```python
from build123d import *

# Parameters (mm, degrees)
F0_R     = 16.3195
F0_R_2   = 0.635
F1_DEPTH = 2.54
F0_R_3   = 20.1295
F2_DEPTH = 19.05


with BuildPart() as f1:
    # F0 (on Top) → F1 (new body)
    with BuildSketch(Plane.XY):
        Circle(F0_R)
        with Locations((-10.644357, -10.906661)):
            Circle(F0_R_2, mode=Mode.SUBTRACT)
        with Locations((-5.567701, -14.186554)):
            Circle(F0_R_2, mode=Mode.SUBTRACT)
        with Locations((-14.003354, -6.013625)):
            Circle(F0_R_2, mode=Mode.SUBTRACT)
        with Locations((-7.184205, -7.184205)):
            Circle(F0_R_2, mode=Mode.SUBTRACT)
        with Locations((-3.888064, -9.386616)):
            Circle(F0_R_2, mode=Mode.SUBTRACT)
        with Locations((-9.388233, -3.884157)):
            Circle(F0_R_2, mode=Mode.SUBTRACT)
        with Locations((-3.592102, -3.592102)):
            Circle(F0_R_2, mode=Mode.SUBTRACT)
        with Locations((-1.944032, -4.693308)):
            Circle(F0_R_2, mode=Mode.SUBTRACT)
        with Locations((-4.694117, -1.942079)):
            Circle(F0_R_2, mode=Mode.SUBTRACT)
        with Locations((0, -15.24)):
            Circle(F0_R_2, mode=Mode.SUBTRACT)
        with Locations((0, -12.7)):
            Circle(F0_R_2, mode=Mode.SUBTRACT)
        with Locations((0, -10.16)):
            Circle(F0_R_2, mode=Mode.SUBTRACT)
        with Locations((6.013625, -14.003354)):
            Circle(F0_R_2, mode=Mode.SUBTRACT)
        with Locations((10.543106, -10.289545)):
            Circle(F0_R_2, mode=Mode.SUBTRACT)
        with Locations((3.982214, -9.347062)):
            Circle(F0_R_2, mode=Mode.SUBTRACT)
        with Locations((0, -7.184205)):
            Circle(F0_R_2, mode=Mode.SUBTRACT)
        with Locations((0, -5.08)):
            Circle(F0_R_2, mode=Mode.SUBTRACT)
        with Locations((7.184205, -7.184205)):
            Circle(F0_R_2, mode=Mode.SUBTRACT)
        with Locations((1.944032, -4.693308)):
            Circle(F0_R_2, mode=Mode.SUBTRACT)
        with Locations((3.592102, -3.592102)):
            Circle(F0_R_2, mode=Mode.SUBTRACT)
        with Locations((4.693308, -1.944032)):
            Circle(F0_R_2, mode=Mode.SUBTRACT)
        with Locations((9.386616, -3.888064)):
            Circle(F0_R_2, mode=Mode.SUBTRACT)
        with Locations((14.186554, -5.567701)):
            Circle(F0_R_2, mode=Mode.SUBTRACT)
        with Locations((-15.24, 0)):
            Circle(F0_R_2, mode=Mode.SUBTRACT)
        with Locations((-12.7, 0)):
            Circle(F0_R_2, mode=Mode.SUBTRACT)
        with Locations((-10.16, 0)):
            Circle(F0_R_2, mode=Mode.SUBTRACT)
        with Locations((-14.124854, 5.548119)):
            Circle(F0_R_2, mode=Mode.SUBTRACT)
        with Locations((-7.184205, 0)):
            Circle(F0_R_2, mode=Mode.SUBTRACT)
        with Locations((-5.08, 0)):
            Circle(F0_R_2, mode=Mode.SUBTRACT)
        with Locations((-9.386616, 3.888064)):
            Circle(F0_R_2, mode=Mode.SUBTRACT)
        with Locations((-4.693308, 1.944032)):
            Circle(F0_R_2, mode=Mode.SUBTRACT)
        with Locations((-3.592102, 3.592102)):
            Circle(F0_R_2, mode=Mode.SUBTRACT)
        with Locations((-1.944032, 4.693308)):
            Circle(F0_R_2, mode=Mode.SUBTRACT)
        with Locations((-7.184205, 7.184205)):
            Circle(F0_R_2, mode=Mode.SUBTRACT)
        with Locations((-3.888064, 9.386616)):
            Circle(F0_R_2, mode=Mode.SUBTRACT)
        with Locations((-10.906661, 10.644357)):
            Circle(F0_R_2, mode=Mode.SUBTRACT)
        with Locations((-6.013625, 14.003354)):
            Circle(F0_R_2, mode=Mode.SUBTRACT)
        Circle(F0_R_2, mode=Mode.SUBTRACT)
        with Locations((1.944032, 4.693308)):
            Circle(F0_R_2, mode=Mode.SUBTRACT)
        with Locations((3.592102, 3.592102)):
            Circle(F0_R_2, mode=Mode.SUBTRACT)
        with Locations((5.08, 0)):
            Circle(F0_R_2, mode=Mode.SUBTRACT)
        with Locations((7.184205, 0)):
            Circle(F0_R_2, mode=Mode.SUBTRACT)
        with Locations((5.04853, 2.09117)):
            Circle(F0_R_2, mode=Mode.SUBTRACT)
        with Locations((0, 5.08)):
            Circle(F0_R_2, mode=Mode.SUBTRACT)
        with Locations((0, 7.184205)):
            Circle(F0_R_2, mode=Mode.SUBTRACT)
        with Locations((3.888064, 9.386616)):
            Circle(F0_R_2, mode=Mode.SUBTRACT)
        with Locations((7.184205, 7.184205)):
            Circle(F0_R_2, mode=Mode.SUBTRACT)
        with Locations((10.16, 0)):
            Circle(F0_R_2, mode=Mode.SUBTRACT)
        with Locations((12.7, 0)):
            Circle(F0_R_2, mode=Mode.SUBTRACT)
        with Locations((10.09706, 4.182339)):
            Circle(F0_R_2, mode=Mode.SUBTRACT)
        with Locations((15.24, 0)):
            Circle(F0_R_2, mode=Mode.SUBTRACT)
        with Locations((14.003354, 6.013625)):
            Circle(F0_R_2, mode=Mode.SUBTRACT)
        with Locations((0, 10.16)):
            Circle(F0_R_2, mode=Mode.SUBTRACT)
        with Locations((0, 12.7)):
            Circle(F0_R_2, mode=Mode.SUBTRACT)
        with Locations((5.567701, 14.186554)):
            Circle(F0_R_2, mode=Mode.SUBTRACT)
        with Locations((0, 15.24)):
            Circle(F0_R_2, mode=Mode.SUBTRACT)
        with Locations((10.644357, 10.906661)):
            Circle(F0_R_2, mode=Mode.SUBTRACT)
    extrude(amount=F1_DEPTH)

    # F0 (on Top) → F2 (join)
    with BuildSketch(Plane.XY):
        Circle(F0_R_3)
        Circle(F0_R, mode=Mode.SUBTRACT)
    extrude(amount=F2_DEPTH)


solid = f1.part
```
Check sheet for the modelled part. Datum: model origin and axes. Units: mm. Give positions to 0.01 mm unless a question says otherwise; leave off trailing zeros. Loops run counter-clockwise (first coordinate to the right, second up) from the corner with the lowest first, then second, coordinate; pieces in that order, holes last. Notation, with made-up numbers: M 67,63 L 104,63 A17 ccw 104,70 Z; hole C 13,-8.75 d9. An arc over 180 degrees is marked long. Answer as CSV lines item,"result".
Item 1: Sectioned sample at A-A, the plane x = -2. Enter the section's corners in (y, z), then the cut area to 3 significant figures.
Reply:
outline,"M -20.03,0 L -5.33,0 L -5.33,2.54 L -16.2,2.54 L -16.2,19.05 L -20.03,19.05 Z; M -4.06,0 L 4.06,0 L 4.06,2.54 L -4.06,2.54 Z; M 5.33,0 L 20.03,0 L 20.03,19.05 L 16.2,19.05 L 16.2,2.54 L 5.33,2.54 Z"
area,"222 mm^2"
Item 2: Sectioned sample at B-B, the plane y = -12.7. Enter the section's corners in (x, z) (3 decimals).
Reply:
outline,"M -15.618,0 L -0.635,0 L -0.635,2.54 L -10.249,2.54 L -10.249,19.05 L -15.618,19.05 Z; M 0.635,0 L 15.618,0 L 15.618,19.05 L 10.249,19.05 L 10.249,2.54 L 0.635,2.54 Z"
Item 3: Scan lines: L1, parallel to Y at x = -10.16, z = 1.4 (3 decimals); L2, parallel to Y at x = 13.5, z = 4.5; L3, parallel to X at y = -0.5, z = 6.75. Record each from-to range of solid material in increasing order.
Reply:
L1,"-17.377 to -11.317, -10.496 to -0.635, 0.635 to 17.377"
L2,"-14.93 to -9.17, 9.17 to 14.93"
L3,"-20.12 to -16.31, 16.31 to 20.12"
Item 4: Depth check by flat-ended pin: pin 1 Ø1.5 at (x, y) = (-7.18, -7.18) entering from +Z; pin 2 Ø5 at (x, z) = (5, 3.5) entering from +Y; pin 3 Ø1 at (y, z) = (11, 6) entering from -X. Enter the tip coordinate at first touch or a pass-through.
Reply:
pin 1,"z = 2.54"
pin 2,"y = 19.97"
pin 3,"x = -17.17"
Item 5: Sectioned sample at D-D, the plane y = 0. State how many separate pieces and enclosed holes the cut face has, then the cut area to 3 significant figures.
Reply:
separate pieces,"12"
enclosed holes,"0"
area,"193 mm^2"
